Could you check a few things on this model? Use its own coordinates, in mm. A direction names the side the tool comes from. Give positions to 0.01 mm unless a question says otherwise; leave off trailing zeros. Order: outer loops, then holes, each group sorted by start corner. A loop starts at its lowest first (then second) coordinate and runs counter-clockwise, first axis right, second up. Notation, with made-up numbers: (26.5, -6.75) - (37.5, -6.75) arc R18 ccw to (37.5, 26.25) - close; hole circle Ø3 at (-16.5, 29.25). An arc over 180 degrees is marked (long way). Put each result on its own line as item: value.
from build123d import *

# Parameters (mm, degrees)
ESQUISSE1_W              = 70
ESQUISSE1_H              = 50
BOSS_EXTRU_1_DEPTH       = 70
ESQUISSE2_R              = 7.75
ENL_V_MAT_EXTRU_1_DEPTH  = 71
ESQUISSE3_R              = 7.75
ENL_V_MAT_EXTRU_2_DEPTH  = 71
ESQUISSE4_W              = 20.2
ESQUISSE4_H              = 20.2
ENL_V_MAT_EXTRU_3_DEPTH  = 51
ESQUISSE7_R              = 11.73674641
ESQUISSE7_R_2            = 5
BOSS_EXTRU_3_DEPTH       = 4
ESQUISSE8_R              = 12.196693844
ESQUISSE8_R_2            = 5
BOSS_EXTRU_4_DEPTH       = 4
ESQUISSE9_W              = 2
ESQUISSE9_H              = 3
ENL_V_MAT_EXTRU_4_DEPTH  = 50.8
ESQUISSE10_W             = 2
ESQUISSE10_H             = 3
ENL_V_MAT_EXTRU_5_DEPTH  = 50.8
ESQUISSE11_W             = 2
ESQUISSE11_H             = 3
ENL_V_MAT_EXTRU_6_DEPTH  = 50.8
ESQUISSE12_W             = 20
ESQUISSE12_H             = 4
BOSS_EXTRU_5_DEPTH       = 12
ESQUISSE13_R             = 1.5
ENL_V_MAT_EXTRU_7_DEPTH  = 36
CONG_1_R                 = 4
ESQUISSE14_W             = 20
ESQUISSE14_H             = 4
BOSS_EXTRU_6_DEPTH       = 12
ESQUISSE15_R             = 1.5
ENL_V_MAT_EXTRU_8_DEPTH  = 36
CONG_3_R                 = 4
ESQUISSE16_W             = 20
ESQUISSE16_H             = 4
BOSS_EXTRU_7_DEPTH       = 12
ESQUISSE17_R             = 1.5
ENL_V_MAT_EXTRU_9_DEPTH  = 20
CONG_4_R                 = 4
ESQUISSE18_W             = 20
ESQUISSE18_H             = 4
BOSS_EXTRU_8_DEPTH       = 12
ESQUISSE19_R             = 1.5
ENL_V_MAT_EXTRU_10_DEPTH = 20
CONG_5_R                 = 4
CONG_6_R                 = 4


with BuildPart() as part:
    # Esquisse1 → Boss.-Extru.1 (new body)
    with BuildSketch(Plane(origin=(0, 0, 0), x_dir=(0, 0, -1), z_dir=(1, 0, 0))):
        with Locations((35, 25)):
            Rectangle(ESQUISSE1_W, ESQUISSE1_H)
    extrude(amount=BOSS_EXTRU_1_DEPTH)

    # Esquisse2 → Enlèv. mat.-Extru.1 (cut, through all)
    with BuildSketch(Plane.XY):
        with Locations((35, 15)):
            Circle(ESQUISSE2_R)
    extrude(amount=-ENL_V_MAT_EXTRU_1_DEPTH, mode=Mode.SUBTRACT)

    # Esquisse3 → Enlèv. mat.-Extru.2 (cut, through all)
    with BuildSketch(Plane.ZY):
        with Locations((-35, 35)):
            Circle(ESQUISSE3_R)
    extrude(amount=-ENL_V_MAT_EXTRU_2_DEPTH, mode=Mode.SUBTRACT)

    # Esquisse4 → Enlèv. mat.-Extru.3 (cut, through all)
    with BuildSketch(Plane.XZ):
        with Locations((10.1, -59.9)):
            Rectangle(ESQUISSE4_W, ESQUISSE4_H)
        with Locations((10.1, -10.1)):
            Rectangle(ESQUISSE4_W, ESQUISSE4_H)
        with Locations((59.9, -10.1)):
            Rectangle(ESQUISSE4_W, ESQUISSE4_H)
        with Locations((59.9, -59.9)):
            Rectangle(ESQUISSE4_W, ESQUISSE4_H)
    extrude(amount=-ENL_V_MAT_EXTRU_3_DEPTH, mode=Mode.SUBTRACT)

    # Esquisse7 → Boss.-Extru.3 (add)
    with BuildSketch(Plane.XY):
        with Locations((35, 15)):
            Circle(ESQUISSE7_R)
        with Locations((35, 15)):
            Circle(ESQUISSE7_R_2, mode=Mode.SUBTRACT)
    extrude(amount=-BOSS_EXTRU_3_DEPTH)

    # Esquisse8 → Boss.-Extru.4 (add)
    with BuildSketch(Plane.ZY):
        with Locations((-35, 35)):
            Circle(ESQUISSE8_R)
        with Locations((-35, 35)):
            Circle(ESQUISSE8_R_2, mode=Mode.SUBTRACT)
    extrude(amount=-BOSS_EXTRU_4_DEPTH)

    # Esquisse9 → Enlèv. mat.-Extru.4 (cut, through all)
    with BuildSketch(Plane.ZY.offset(-20.2)):
        with Locations((-69, 4.5)):
            Rectangle(ESQUISSE9_W, ESQUISSE9_H)
    extrude(amount=-ENL_V_MAT_EXTRU_4_DEPTH, mode=Mode.SUBTRACT)

    # Esquisse10 → Enlèv. mat.-Extru.5 (cut, through all)
    with BuildSketch(Plane(origin=(0, 0, -49.8), x_dir=(-1, 0, 0), z_dir=(0, 0, -1))):
        with Locations((-1, 4.5)):
            Rectangle(ESQUISSE10_W, ESQUISSE10_H)
    extrude(amount=-ENL_V_MAT_EXTRU_5_DEPTH, mode=Mode.SUBTRACT)

    # Esquisse11 → Enlèv. mat.-Extru.6 (cut, through all)
    with BuildSketch(Plane(origin=(0, 0, -49.8), x_dir=(-1, 0, 0), z_dir=(0, 0, -1))):
        with Locations((-69, 4.5)):
            Rectangle(ESQUISSE11_W, ESQUISSE11_H)
    extrude(amount=-ENL_V_MAT_EXTRU_6_DEPTH, mode=Mode.SUBTRACT)

    # Esquisse12 → Boss.-Extru.5 (add)
    with BuildSketch(Plane.ZY):
        with Locations((-35, 17)):
            Rectangle(ESQUISSE12_W, ESQUISSE12_H)
    extrude(amount=BOSS_EXTRU_5_DEPTH)

    # Esquisse13 → Enlèv. mat.-Extru.7 (cut, through all)
    with BuildSketch(Plane.XZ.offset(-15)):
        with Locations(Location((-8, -30, 0), (0, 0, 270))):  # turned: the seam where the file's is
            Circle(ESQUISSE13_R)
        with Locations(Location((-8, -40, 0), (0, 0, 270))):  # turned: the seam where the file's is
            Circle(ESQUISSE13_R)
    extrude(amount=-ENL_V_MAT_EXTRU_7_DEPTH, mode=Mode.SUBTRACT)

    # Congé1
    cong_1_edges = [part.edges().sort_by_distance(p)[0] for p in [
        (-12, 17, -25),
        (-12, 17, -45),
    ]]
    fillet(cong_1_edges, radius=CONG_1_R)

    # Esquisse14 → Boss.-Extru.6 (add)
    with BuildSketch(Plane(origin=(70, 0, 0), x_dir=(0, 0, -1), z_dir=(1, 0, 0))):
        with Locations((35, 17)):
            Rectangle(ESQUISSE14_W, ESQUISSE14_H)
    extrude(amount=BOSS_EXTRU_6_DEPTH)

    # Esquisse15 → Enlèv. mat.-Extru.8 (cut, through all)
    with BuildSketch(Plane.XZ.offset(-15)):
        with Locations(Location((78, -40, 0), (0, 0, 270))):  # turned: the seam where the file's is
            Circle(ESQUISSE15_R)
        with Locations(Location((78, -30, 0), (0, 0, 270))):  # turned: the seam where the file's is
            Circle(ESQUISSE15_R)
    extrude(amount=-ENL_V_MAT_EXTRU_8_DEPTH, mode=Mode.SUBTRACT)

    # Congé3
    cong_3_edges = [part.edges().sort_by_distance(p)[0] for p in [
        (82, 17, -45),
        (82, 17, -25),
    ]]
    fillet(cong_3_edges, radius=CONG_3_R)

    # Esquisse16 → Boss.-Extru.7 (add)
    with BuildSketch(Plane.XY):
        with Locations((35, 33)):
            Rectangle(ESQUISSE16_W, ESQUISSE16_H)
    extrude(amount=BOSS_EXTRU_7_DEPTH)

    # Esquisse17 → Enlèv. mat.-Extru.9 (cut, through all)
    with BuildSketch(Plane.XZ.offset(-31)):
        with Locations((40, 8)):
            Circle(ESQUISSE17_R)
        with Locations((30, 8)):
            Circle(ESQUISSE17_R)
    extrude(amount=-ENL_V_MAT_EXTRU_9_DEPTH, mode=Mode.SUBTRACT)

    # Congé4
    cong_4_edges = [part.edges().sort_by_distance(p)[0] for p in [
        (45, 33, 12),
        (25, 33, 12),
    ]]
    fillet(cong_4_edges, radius=CONG_4_R)

    # Esquisse18 → Boss.-Extru.8 (add)
    with BuildSketch(Plane(origin=(0, 0, -70), x_dir=(-1, 0, 0), z_dir=(0, 0, -1))):
        with Locations((-35, 33)):
            Rectangle(ESQUISSE18_W, ESQUISSE18_H)
    extrude(amount=BOSS_EXTRU_8_DEPTH)

    # Esquisse19 → Enlèv. mat.-Extru.10 (cut, through all)
    with BuildSketch(Plane.XZ.offset(-31)):
        with Locations((30, -78)):
            Circle(ESQUISSE19_R)
        with Locations((40, -78)):
            Circle(ESQUISSE19_R)
    extrude(amount=-ENL_V_MAT_EXTRU_10_DEPTH, mode=Mode.SUBTRACT)

    # Congé5
    cong_5_edges = [part.edges().sort_by_distance(p)[0] for p in [
        (25, 33, -82),
        (45, 33, -82),
    ]]
    fillet(cong_5_edges, radius=CONG_5_R)

    # Congé6
    cong_6_edges = [part.edges().sort_by_distance(p)[0] for p in [
        (0, 19, -35),
        (70, 19, -35),
        (35, 35, 0),
        (35, 35, -70),
    ]]
    fillet(cong_6_edges, radius=CONG_6_R)


solid = part.part
1) Suppose I cut it at B-B, the plane x = 54.5. List the corners of the cut face in (y, z) for me, and give its area (3 significant figures).
Filled in:
outline: (0, -49.8) - (50, -49.8) - (50, -20.2) - (0, -20.2) - close; hole circle Ø15.5 at (35, -35)
area: 1,290 mm^2
2) If I drill on line 1 (X direction, y = 32, z = -78); line 2 (Z direction, x = 40, y = 32); line 3 (Z direction, x = 30, y = 33), over which ranges is the centre line in solid material (lowest first)? Write a range as [from, to].
Filled in:
line 1: x = [25, 28.5], [31.5, 38.5], [41.5, 45]
line 2: z = [-82, -79.5], [-76.5, -42.15], [-27.85, 6.5], [9.5, 12]
line 3: z = [-82, -79.5], [-76.5, -42.49], [-27.51, 6.5], [9.5, 12]
3) I'm going to push flat-ended pins straight in: pin 1 (1.5 mm diameter, centred on y = 2, z = -30, fed in from +X); pin 2 (3.5 mm diameter, centred on x = 30, z = 8, fed in from -Y); pin 3 (9.5 mm diameter, centred on x = -6, z = -31, fed in from -Y); pin 4 (23.5 mm diameter, centred on y = 28.5, z = -36.5, fed in from -X). Where does each tip first touch, or does it pass through?
Filled in:
pin 1: stops at x = 70
pin 2: stops at y = 31
pin 3: stops at y = 15
pin 4: stops at x = -12
4) Which directions (+Z, -Z, +X, -X, +Y, -Y) give clear straight access to the entire face, cutting with the end or side of a thin tool? Please do faces 1 (the flat face through (78, 19, -35)), 2 (the flat face through (35, 31, 6)), 3 (the flat face through (76, 15, -35)), 4 (the flat face through (35, 31, -76)).
Filled in:
face 1: +Z, -Z, +X, +Y
face 2: +Z, +X, -X, -Y
face 3: +Z, -Z, +X, -Y
face 4: -Z, +X, -X, -Y
5) Suppose I cut it at C-C, the plane y = 12.5. List the corners of the cut face in (x, z) for me.
Filled in:
outline: (0, -49.8) - (20.2, -49.8) - (20.2, -70) - (27.66, -70) - (27.66, -4) - (30.67, -4) - (30.67, 0) - (20.2, 0) - (20.2, -20.2) - (0, -20.2) - close; (39.33, -4) - (42.34, -4) - (42.34, -70) - (49.8, -70) - (49.8, -49.8) - (70, -49.8) - (70, -20.2) - (49.8, -20.2) - (49.8, 0) - (39.33, 0) - close
6) We'd pull the mould along X, two halves only. Please class faces 5 (the flat face through (-12, 17, -35)), 6 (the cylindrical face through (43.859, 33.028, -80.797)), 7 (the flat face through (35, 28, -70)), 8 (the cylindrical face through (-7.93, 16.97, -28.5)): pulls with the +X half, pulls with the -X half, needs draft (parallel to the pull), parting line crosses it, or undercut.
Filled in:
face 5: pulls with the -X half
face 6: pulls with the +X half
face 7: needs draft
face 8: undercut
7) Suppose I cut it at D-D, the plane y = 44. List the corners of the cut face in (x, z) for me.
Filled in:
outline: (0, -49.8) - (20.2, -49.8) - (20.2, -70) - (49.8, -70) - (49.8, -49.8) - (70, -49.8) - (70, -20.2) - (49.8, -20.2) - (49.8, 0) - (20.2, 0) - (20.2, -20.2) - (0, -20.2) - close
8) Suppose I cut it at A-A, the plane z = -22.5. List the corners of the cut face in (x, y) for me.
Filled in:
outline: (0, 0) - (70, 0) - (70, 3) - (68, 3) - (68, 6) - (70, 6) - (70, 50) - (0, 50) - (0, 6) - (2, 6) - (2, 3) - (0, 3) - close; hole circle Ø15.5 at (35, 15)
